CAD build for the part. Positions are in the model's coordinates, mm. Face numbers are marked on the shaded views. Give positions to 0.01 mm unless a question says otherwise; leave off trailing zeros. Order: outer loops, then holes, each group sorted by start corner. A loop starts at its lowest first (then second) coordinate and runs counter-clockwise, first axis right, second up. Notation, with made-up numbers: M 18,13.25 L 74,13.25 A8 ccw 74,26.25 Z; hole C 75.5,56 d8. An arc over 180 degrees is marked long. Put each result on its own line as item: value. Start each with the question number.
1) Cut at C-C (y = -4.5). Write the cut outline in (x, z).
2) Cut at B-B (z = 5). Write the cut outline in (x, y), and give its area (3 significant figures).
3) Cut at D-D (x = 123.5). Write the cut outline in (y, z).
4) Cut at A-A (x = -3). Write the cut outline in (y, z), and give its area (3 significant figures).
5) Pin check, flat tips, straight feed: pin 1 (6 mm diameter, centred on y = 11, z = 3, fed in from +X); pin 2 (3 mm diameter, centred on y = -19.5, z = 2.5, fed in from +X); pin 3 (2 mm diameter, centred on y = 11, z = 2.5, fed in from -X). Stop position of each tip, or through.
6) Drill centre lines: line 1 (Y direction, x = 127, z = 8.75); line 2 (Y direction, x = 134, z = 8); line 3 (X direction, y = -11, z = 6.5). Where is each one in solid material? Low to high. Write a range as [from, to].
7) Two-plate mould, pull along Y, no slides. Class the marked faces 1, 2, 3 and 4: released by +Y, released by -Y, zero draft, split by the parting line, or undercut.
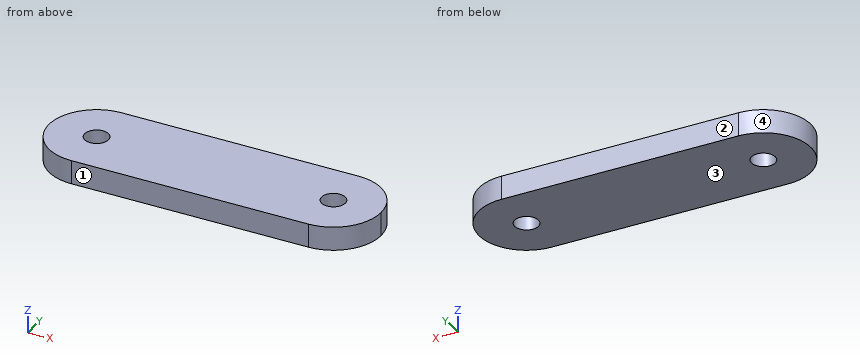
```python
from build123d import *

# Parameters (mm, degrees)
F2_DEPTH = 12.7
F3_D     = 12.7
F3_DEPTH = 25.4
F4_D     = 12.7
F4_DEPTH = 127


with BuildPart() as f2:
    # F0 (on Top) → F2 (new body)
    with BuildSketch(Plane.XY):
        with BuildLine():
            ThreePointArc((25.4, 0), (17.960512, -17.960512), (0, -25.4))
            Line((0, -25.4), (127, -25.4))
            ThreePointArc((127, -25.4), (101.6, 0), (127, 25.4))
            Line((127, 25.4), (0, 25.4))
            ThreePointArc((0, 25.4), (17.960512, 17.960512), (25.4, 0))
        make_face()
        with BuildLine():
            ThreePointArc((0, 25.4), (-25.4, 0), (0, -25.4))
            ThreePointArc((0, -25.4), (17.960512, -17.960512), (25.4, 0))
            ThreePointArc((25.4, 0), (17.960512, 17.960512), (0, 25.4))
        make_face()
        with BuildLine():
            ThreePointArc((127, 25.4), (101.6, 0), (127, -25.4))
            ThreePointArc((127, -25.4), (144.960512, -17.960512), (152.4, 0))
            ThreePointArc((152.4, 0), (144.960512, 17.960512), (127, 25.4))
        make_face()
    extrude(amount=F2_DEPTH)

    # F3
    with Locations(Plane(origin=(0, 0, 0), x_dir=(1, 0, 0), z_dir=(0, 0, -1))):
        with Locations((0, 0)):
            Hole(F3_D / 2, depth=F3_DEPTH)

    # F4
    with Locations(Plane(origin=(0, 0, 0), x_dir=(1, 0, 0), z_dir=(0, 0, -1))):
        with Locations((127, 0)):
            Hole(F4_D / 2, depth=F4_DEPTH)


solid = f2.part
```
Solution:
1. outline: M -25,0 L -4.48,0 L -4.48,12.7 L -25,12.7 Z; M 4.48,0 L 122.52,0 L 122.52,12.7 L 4.48,12.7 Z; M 131.48,0 L 152,0 L 152,12.7 L 131.48,12.7 Z
2. outline: M 0,-25.4 L 127,-25.4 A25.4 ccw 152.4,0 A25.4 ccw 127,25.4 L 0,25.4 A25.4 ccw Z; hole C 0,0 d12.7; hole C 127,0 d12.7
2. area: 8,230 mm²
3. outline: M -25.4,0 L -5.3,0 L -5.3,12.7 L -25.4,12.7 Z; M 5.3,0 L 25.4,0 L 25.4,12.7 L 5.3,12.7 Z
4. outline: M -25.22,0 L -5.6,0 L -5.6,12.7 L -25.22,12.7 Z; M 5.6,0 L 25.22,0 L 25.22,12.7 L 5.6,12.7 Z
4. area: 498 mm²
5. pin 1: x = 151.11
5. pin 2: x = 144.92
5. pin 3: x = -23.35
6. line 1: [-25.4, -6.35], [6.35, 25.4]
6. line 2: [-24.42, 24.42]
6. line 3: [-22.89, 149.89]
7. face 1: released by -Y
7. face 2: released by +Y
7. face 3: zero draft
7. face 4: split by the parting line
